Could you check a few things on this model? Use its own coordinates, in mm. Face numbers are marked on the shaded views. A direction names the side the tool comes from. Round coordinates to 2 decimals unless told otherwise and drop trailing zeros. Loops run counter-clockwise (first coordinate to the right, second up) from the corner with the lowest first, then second, coordinate; pieces in that order, holes last.
from build123d import *

# Parameters (mm, degrees)
SKETCH001_R           = 57.15
SKETCH001_R_2         = 52.15
EXTRUDE001_DEPTH      = 360
EXTRUDE002_DEPTH      = 5
ARRAY_COUNT           = 4
ARRAY_PLACEMENT_ANGLE = 45
EXTRUDE003_DEPTH      = 20
SKETCH_W              = 260
SKETCH_H              = 260
SKETCH_R              = 7
EXTRUDE_DEPTH         = 20


with BuildPart() as r114x5:
    # Sketch001 (on Face10 of Extrude) → Extrude001 (new body)
    with BuildSketch(Plane.XY.offset(20)):
        Circle(SKETCH001_R)
        Circle(SKETCH001_R_2, mode=Mode.SUBTRACT)
    extrude(amount=EXTRUDE001_DEPTH)


with BuildPart() as obj1:
    # Sketch002 → Extrude002 (new body, symmetric)
    with BuildSketch(Plane.XZ):
        Polygon((54.65, 160), (77.15, 160), (119.65, 40), (119.65, 20), (74.65, 20), (54.65, 40), align=None)
    extrude(amount=EXTRUDE002_DEPTH, both=True)

    # Array: obj1 ×4 about axis
    array_axis = Axis((0, 0, 0), (0, 0, 1))


with BuildPart() as obj1_1:
    add(obj1.part)
    for i in range(1, ARRAY_COUNT):
        add(obj1.part.rotate(array_axis, i * 360 / ARRAY_COUNT))


with BuildPart() as obj1_2:
    # Array placement: moved
    add(obj1_1.part.rotate(Axis((0, 0, 0), (0, 0, 1)), ARRAY_PLACEMENT_ANGLE))


with BuildPart() as lastplatte:
    # Sketch003 (on Face4 of Extrude001) → Extrude003 (new body)
    with BuildSketch(Plane.XY.offset(380)):
        Polygon((72.49808, -19.425802), (53.072278, 53.072278), (-19.425802, 72.49808), (-72.49808, 19.425802), (-53.072278, -53.072278), (19.425802, -72.49808), align=None)
    extrude(amount=EXTRUDE003_DEPTH)


with BuildPart() as fusion:
    # Sketch → Extrude (new body)
    with BuildSketch(Plane.XY):
        Rectangle(SKETCH_W, SKETCH_H)
        with Locations((-105, 105)):
            Circle(SKETCH_R, mode=Mode.SUBTRACT)
        with Locations((105, 105)):
            Circle(SKETCH_R, mode=Mode.SUBTRACT)
        with Locations((-105, -105)):
            Circle(SKETCH_R, mode=Mode.SUBTRACT)
        with Locations((105, -105)):
            Circle(SKETCH_R, mode=Mode.SUBTRACT)
    extrude(amount=EXTRUDE_DEPTH)

    # Fusion: union R114x5, obj1, lastplatte
    add(r114x5.part)
    add(obj1_2.part)
    add(lastplatte.part)


solid = fusion.part
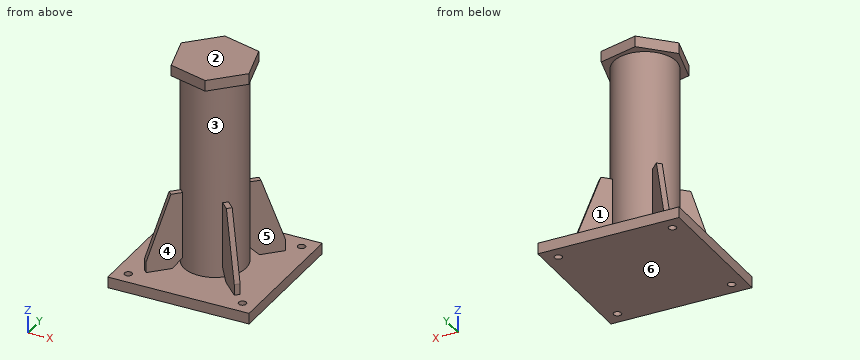
Item 1: Will these pins go through, and if not, where does the flat tip stop? pin 1 (22.5 mm diameter, centred on x = -105, y = -105, fed in from +Z); pin 2 (8 mm diameter, centred on y = 29.5, z = 136.5, fed in from +X); pin 3 (8.5 mm diameter, centred on x = -105, y = 105, fed in from -Z); pin 4 (6 mm diameter, centred on x = -27.5, z = 306.5, fed in from +Y).
Results list:
pin 1: stops at z = 20
pin 2: stops at x = 51.15
pin 3: passes through
pin 4: stops at y = 51.63
Item 2: If I drill on line 1 along Y through (x, z) = (-105, 13); line 2 along Z through (x, y) = (-36.5, -47.5); line 3 along Y through (x, z) = (0, 227.5), over which ranges is the centre line in solid material (lowest first)?
Results list:
line 1: y = -130 to -112, -98 to 98, 112 to 130
line 2: z = 0 to 20, 380 to 400
line 3: y = -57.15 to -52.15, 52.15 to 57.15
Item 3: For the marked faces 1, 2 and 3, which set-ups out of +Z, -Z, +X, -X, +Y, -Y let a thin tool reach every point of the face, with its end or its side?
Results list:
face 1: +Y
face 2: +Z, +X, -X, +Y, -Y
face 3: none
Item 4: If we section it at A-A, the plane y = 105: Please give me the cut outline in (x, z).
Results list:
outline: (-130, 0) - (-112, 0) - (-112, 20) - (-130, 20) - close; (-98, 0) - (98, 0) - (98, 20) - (-98, 20) - close; (112, 0) - (130, 0) - (130, 20) - (112, 20) - close
Item 5: If we section it at C-C, the plane z = 56.5: Please give me the cut outline in (x, y).
Results list:
outline: (-84.01, -76.94) - (-76.94, -84.01) - (-36.72, -43.79) arc R57.15 ccw to (36.72, -43.79) - (76.94, -84.01) - (84.01, -76.94) - (43.79, -36.72) arc R57.15 ccw to (43.79, 36.72) - (84.01, 76.94) - (76.94, 84.01) - (36.72, 43.79) arc R57.15 ccw to (-36.72, 43.79) - (-76.94, 84.01) - (-84.01, 76.94) - (-43.79, 36.72) arc R57.15 ccw to (-43.79, -36.72) - close; hole circle Ø104.3 at (0, 0)
Item 6: If we section it at D-D, the plane x = 0: Please give me the cut outline in (y, z), then the cut area to 3 significant figures.
Results list:
outline: (-130, 0) - (130, 0) - (130, 20) - (57.15, 20) - (57.15, 380) - (67.29, 380) - (67.29, 400) - (-67.29, 400) - (-67.29, 380) - (-57.15, 380) - (-57.15, 20) - (-130, 20) - close; hole (-52.15, 20) - (52.15, 20) - (52.15, 380) - (-52.15, 380) - close
area: 11,500 mm2
Item 7: We'd pull the mould along Y, two halves only. Please class the marked faces 4, 5 and 6: released by +Y, released by -Y, zero draft, split by the parting line, or undercut.
Results list:
face 4: released by -Y
face 5: undercut
face 6: zero draft
